Verification items for this drawing (mm, ordinates from the low corner). Round coordinates to 2 decimals unless told otherwise and drop trailing zeros. Order: outer loops, then holes, each group sorted by start corner. A loop starts at its lowest first (then second) coordinate and runs counter-clockwise, first axis right, second up.
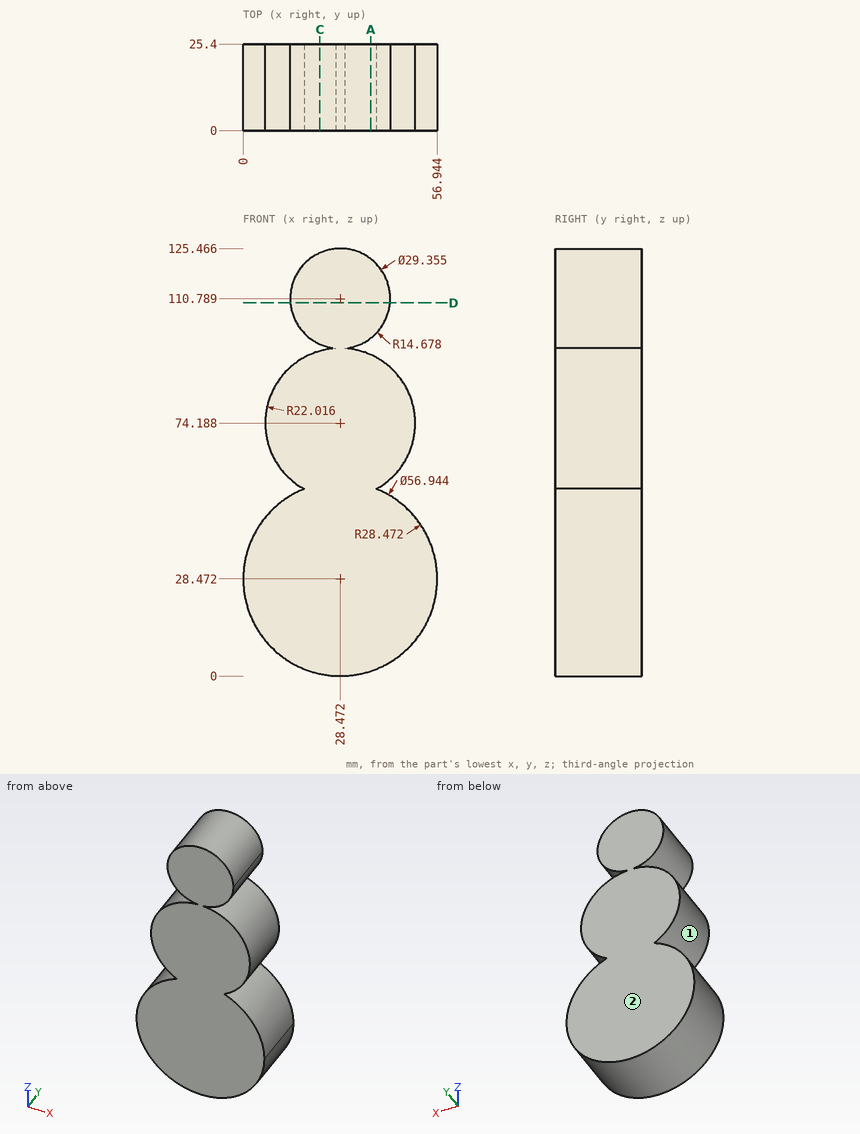
Item 1: Sectioned sample at A-A (x = 37.5). Record the cut outline in (y, z), and give its area (4 significant figures).
Answer:
outline: (0, 1.47) - (25.4, 1.47) - (25.4, 94.27) - (0, 94.27) - close; (0, 99.22) - (25.4, 99.22) - (25.4, 122.36) - (0, 122.36) - close
area: 2,945 mm2
Item 2: Sectioned sample at C-C (x = 22.5). Record the cut outline in (y, z).
Answer:
outline: (0, 0.63) - (25.4, 0.63) - (25.4, 95.38) - (0, 95.38) - close; (0, 97.38) - (25.4, 97.38) - (25.4, 124.2) - (0, 124.2) - close
Item 3: Release check for a two-part mould opening along Z. For the marked faces 1 and 2 record: released by +Z, released by -Z, zero draft, split by the parting line, or undercut.
Answer:
face 1: undercut
face 2: zero draft
Item 4: Scan lines: line 1 along Z through (x, y) = (42, 14.25) (1 decimal); line 2 along Z through (x, y) = (36.5, 21) (1 decimal); line 3 along Z through (x, y) = (20.5, 17.25) (1 decimal). Record each from-to range of solid material in increasing order.
Answer:
line 1: z = 3.4 to 53.5, 56.8 to 91.6, 105.1 to 116.5
line 2: z = 1.2 to 94.7, 98.5 to 123.1
line 3: z = 1.1 to 94.7, 98.5 to 123.1
Item 5: Go/stop test with flat-tipped pins: P1, Ø10, axis at y = 22.5, z = 23, coming from the +X side; P2, Ø2, axis at y = 15, z = 13.5, coming from the +X side; P3, Ø6, axis at x = 40, y = 5.5, coming from the +Z side (1 decimal). Record where each tip stops, or that it passes through.
Answer:
P1: stops at x = 56.94
P2: stops at x = 53.28
P3: stops at z = 122.7
Item 6: Sectioned sample at D-D (z = 109.5). Record the cut outline in (x, y), and give its area (3 significant figures).
Answer:
outline: (13.85, 0) - (43.09, 0) - (43.09, 25.4) - (13.85, 25.4) - close
area: 743 mm2
